Build history of the part. All positions in model axes, mm. Face numbers are marked on the shaded views. Give positions to 0.01 mm unless a question says otherwise; leave off trailing zeros. Loops run counter-clockwise (first coordinate to the right, second up) from the corner with the lowest first, then second, coordinate; pieces in that order, holes last. Notation, with made-up numbers: M 19,20.25 L 61,20.25 A30 ccw 61,48.25 Z; hole C -39,-14.5 d6. An arc over 180 degrees is marked long. Put each result on its own line as item: value.
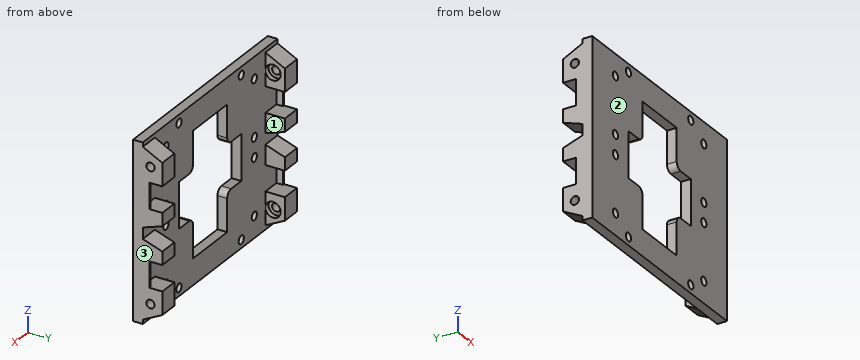
```python
from build123d import *

# Parameters (mm, degrees)
SKETCH1_W                    = 85.09
SKETCH1_H                    = 68.58
BOSS_EXTRUDE1_DEPTH          = 5.08
F_30_0_1285_DIAMETER_HOLE1_D = 3.2639
SKETCH3_W                    = 31.877
SKETCH3_H                    = 68.58
SKETCH3_W_2                  = 53.213
CUT_EXTRUDE1_DEPTH           = 1.27
F_30_0_1285_DIAMETER_HOLE2_D = 3.2639
BOSS_EXTRUDE2_DEPTH          = 7.62
SKETCH10_W                   = 10
SKETCH10_H                   = 2.54
BOSS_EXTRUDE3_DEPTH          = 0.635
BOSS_EXTRUDE4_DEPTH          = 7.62
SKETCH12_W                   = 10
SKETCH12_H                   = 2.54
BOSS_EXTRUDE5_DEPTH          = 0.635
SKETCH13_W                   = 21.59
SKETCH13_H                   = 15.24
SKETCH13_W_2                 = 8.89
SKETCH13_H_2                 = 17.78
CUT_EXTRUDE3_DEPTH           = 4.81
FILLET1_R                    = 2.54
CUT_EXTRUDE4_START           = -7.62
SKETCH14_R                   = 1.63195
CUT_EXTRUDE4_DEPTH           = 8.62
CUT_EXTRUDE4_DEPTH_BACK      = 86.09
CUT_EXTRUDE5_START           = -7.62
SKETCH14_3_R                 = 3
SKETCH14_3_R_2               = 1.63195
CUT_EXTRUDE5_DEPTH           = 2
CUT_EXTRUDE6_START           = -77.47
SKETCH14_4_R                 = 3
SKETCH14_4_R_2               = 1.63195
CUT_EXTRUDE6_DEPTH           = 2


with BuildPart() as part:
    # Sketch1 → Boss-Extrude1 (new body)
    with BuildSketch(Plane(origin=(0, 0, 0), x_dir=(1, 0, 0), z_dir=(0, 1, 0))):
        with Locations((42.545, 34.29)):
            Rectangle(SKETCH1_W, SKETCH1_H)
    extrude(amount=BOSS_EXTRUDE1_DEPTH)

    # #30 (0.1285) Diameter Hole1 (through all)
    with Locations(Plane(origin=(62.23, 5.08, -65.405), x_dir=(0, 0, 1), z_dir=(0, 1, 0))):
        with Locations((0, 0), (0, -39.37), (62.23, -39.37), (62.23, 0)):
            Hole(F_30_0_1285_DIAMETER_HOLE1_D / 2)

    # Sketch3 → Cut-Extrude1 (cut)
    with BuildSketch(Plane(origin=(0, 5.08, 0), x_dir=(1, 0, 0), z_dir=(0, 1, 0))):
        with Locations((69.1515, 34.29)):
            Rectangle(SKETCH3_W, SKETCH3_H)
        with Locations((26.6065, 34.29)):
            Rectangle(SKETCH3_W_2, SKETCH3_H)
    extrude(amount=-CUT_EXTRUDE1_DEPTH, mode=Mode.SUBTRACT)

    # #30 (0.1285) Diameter Hole2 (through all)
    with Locations(Plane(origin=(70.455, 3.81, -38.1), x_dir=(0, 0, 1), z_dir=(0, 1, 0))):
        with Locations((0, 0), (-22.098, 0), (7.62, 0), (29.718, 0), (29.718, -55.82), (7.62, -55.82), (0, -55.82), (-22.098, -55.82)):
            Hole(F_30_0_1285_DIAMETER_HOLE2_D / 2)

    # Sketch9 → Boss-Extrude2 (add)
    with BuildSketch(Plane.ZY):
        Polygon((-14.431, 3.81), (-1.651, 3.81), (-5.541, 11.43), (-14.431, 11.43), align=None)
        Polygon((-24.431, 3.81), (-24.431, 11.43), (-29.511, 11.43), (-32.131, 3.81), align=None)
        Polygon((-44.149, 3.81), (-44.149, 11.43), (-39.069, 11.43), (-36.449, 3.81), align=None)
        Polygon((-54.149, 3.81), (-54.149, 11.43), (-63.039, 11.43), (-66.929, 3.81), align=None)
    extrude(amount=-BOSS_EXTRUDE2_DEPTH)

    # Sketch10 → Boss-Extrude3 (add)
    with BuildSketch(Plane.ZY):
        with Locations((-49.149, 5.08)):
            Rectangle(SKETCH10_W, SKETCH10_H)
        with Locations((-19.431, 5.08)):
            Rectangle(SKETCH10_W, SKETCH10_H)
    extrude(amount=-BOSS_EXTRUDE3_DEPTH)

    # Sketch11 → Boss-Extrude4 (add)
    with BuildSketch(Plane(origin=(85.09, 0, 0), x_dir=(0, 0, -1), z_dir=(1, 0, 0))):
        Polygon((24.431, 3.81), (24.431, 11.43), (29.511, 11.43), (32.11195, 3.81), align=None)
        Polygon((44.149, 3.81), (44.149, 11.43), (39.069, 11.43), (36.46805, 3.81), align=None)
        Polygon((14.431, 11.43), (14.431, 3.81), (1.651, 3.81), (5.541, 11.43), align=None)
        Polygon((63.039, 11.43), (66.929, 3.81), (54.149, 3.81), (54.149, 11.43), align=None)
    extrude(amount=-BOSS_EXTRUDE4_DEPTH)

    # Sketch12 → Boss-Extrude5 (add)
    with BuildSketch(Plane(origin=(85.09, 0, 0), x_dir=(0, 0, -1), z_dir=(1, 0, 0))):
        with Locations((19.431, 5.08)):
            Rectangle(SKETCH12_W, SKETCH12_H)
        with Locations((49.149, 5.08)):
            Rectangle(SKETCH12_W, SKETCH12_H)
    extrude(amount=-BOSS_EXTRUDE5_DEPTH)

    # Sketch13 → Cut-Extrude3 (cut, through all)
    with BuildSketch(Plane(origin=(0, 3.81, 0), x_dir=(1, 0, 0), z_dir=(0, 1, 0))):
        with Locations((42.545, 50.8)):
            Rectangle(SKETCH13_W, SKETCH13_H)
        with Locations((27.305, 34.29)):
            Rectangle(SKETCH13_W_2, SKETCH13_H_2)
        with Locations((42.545, 34.29)):
            Rectangle(SKETCH13_W, SKETCH13_H_2)
        with Locations((57.785, 34.29)):
            Rectangle(SKETCH13_W_2, SKETCH13_H_2)
        with Locations((42.545, 17.78)):
            Rectangle(SKETCH13_W, SKETCH13_H)
    extrude(amount=-CUT_EXTRUDE3_DEPTH, mode=Mode.SUBTRACT)

    # Fillet1
    fillet1_edges = [part.edges().sort_by_distance(p)[0] for p in [
        (31.75, 1.905, -43.18),
        (53.34, 1.905, -43.18),
        (53.34, 1.905, -25.4),
        (31.75, 1.905, -25.4),
    ]]
    fillet(fillet1_edges, radius=FILLET1_R)

    # Sketch14 → Cut-Extrude4 (cut, two sides)
    with BuildSketch(Plane(origin=(85.09, 0, 0), x_dir=(0, 0, -1), z_dir=(1, 0, 0)).offset(CUT_EXTRUDE4_START)) as cut_extrude4_sk:
        with Locations((8.382, 6.81)):
            Circle(SKETCH14_R)
        with Locations((60.198, 6.81)):
            Circle(SKETCH14_R)
    extrude(amount=CUT_EXTRUDE4_DEPTH, mode=Mode.SUBTRACT)
    extrude(cut_extrude4_sk.sketch, amount=-CUT_EXTRUDE4_DEPTH_BACK, mode=Mode.SUBTRACT)

    # Sketch14<3> → Cut-Extrude5 (cut)
    with BuildSketch(Plane(origin=(85.09, 0, 0), x_dir=(0, 0, -1), z_dir=(1, 0, 0)).offset(CUT_EXTRUDE5_START)):
        with Locations((8.382, 6.81)):
            Circle(SKETCH14_3_R)
        with Locations((8.382, 6.81)):
            Circle(SKETCH14_3_R_2, mode=Mode.SUBTRACT)
        with Locations((60.198, 6.81)):
            Circle(SKETCH14_3_R)
        with Locations((60.198, 6.81)):
            Circle(SKETCH14_3_R_2, mode=Mode.SUBTRACT)
    extrude(amount=CUT_EXTRUDE5_DEPTH, mode=Mode.SUBTRACT)

    # Sketch14<4> → Cut-Extrude6 (cut)
    with BuildSketch(Plane(origin=(85.09, 0, 0), x_dir=(0, 0, -1), z_dir=(1, 0, 0)).offset(CUT_EXTRUDE6_START)):
        with Locations((8.382, 6.81)):
            Circle(SKETCH14_4_R)
        with Locations((8.382, 6.81)):
            Circle(SKETCH14_4_R_2, mode=Mode.SUBTRACT)
        with Locations((60.198, 6.81)):
            Circle(SKETCH14_4_R)
        with Locations((60.198, 6.81)):
            Circle(SKETCH14_4_R_2, mode=Mode.SUBTRACT)
    extrude(amount=-CUT_EXTRUDE6_DEPTH, mode=Mode.SUBTRACT)


solid = part.part
```
Q1. Slice it at C-C (z = -38.1). List the corners of the cut face in (x, y).
Here are the results:
outline: M 0,0 L 13,0 L 13,3.81 L 7.62,3.81 L 7.62,8.61 L 0,8.61 Z; M 16.27,0 L 22.86,0 L 22.86,3.81 L 16.27,3.81 Z; M 62.23,0 L 68.82,0 L 68.82,3.81 L 62.23,3.81 Z; M 72.09,0 L 85.09,0 L 85.09,8.59 L 77.47,8.59 L 77.47,3.81 L 72.09,3.81 Z
Q2. Mould opens along X. For the marked faces 1, 2 and 3 say: pulls with the +X half, pulls with the -X half, needs draft (parallel to the pull), parting line crosses it, or undercut.
Here are the results:
face 1: undercut
face 2: needs draft
face 3: pulls with the +X half
Q3. Probe line 1 (Z direction, x = 50, y = 1.5); line 2 (Z direction, x = 28.5, y = 2); line 3 (Z direction, x = 78, y = 9.5). List the from-to ranges inside material, lowest first. Write a range as from..to.
Here are the results:
line 1: -68.58..-58.42, -10.16..0
line 2: -68.58..-43.18, -25.4..0
line 3: -64.02..-61.53, -58.87..-54.15, -44.15..-38.41, -30.17..-24.43, -14.43..-9.71, -7.05..-4.56
Q4. Drop flat-ended pins along their axis: pin 1 Ø6 at (y, z) = (9.5, -50.5) entering from +X; pin 2 Ø1.5 at (x, z) = (70, -13.5) entering from +Y; pin 3 Ø4 at (x, y) = (82, 7) entering from +Z. Give the stop position or say it passes through.
Here are the results:
pin 1: through
pin 2: y = 3.81
pin 3: z = -2.26
Q5. Slice it at A-A (z = -52). List the corners of the cut face in (x, y) (3 decimals), and give its area (3 significant figures).
Here are the results:
outline: M 0,0 L 31.75,0 L 31.75,3.81 L 0.635,3.81 L 0.635,6.35 L 0,6.35 Z; M 53.34,0 L 85.09,0 L 85.09,6.35 L 84.455,6.35 L 84.455,3.81 L 53.34,3.81 Z
area: 245 mm²
Q6. Slice it at B-B (x = 48). List the corners of the cut face in (y, z), and give its area (3 significant figures).
Here are the results:
outline: M 0,-68.58 L 3.81,-68.58 L 3.81,-58.42 L 0,-58.42 Z; M 0,-10.16 L 3.81,-10.16 L 3.81,0 L 0,0 Z
area: 77.4 mm²
